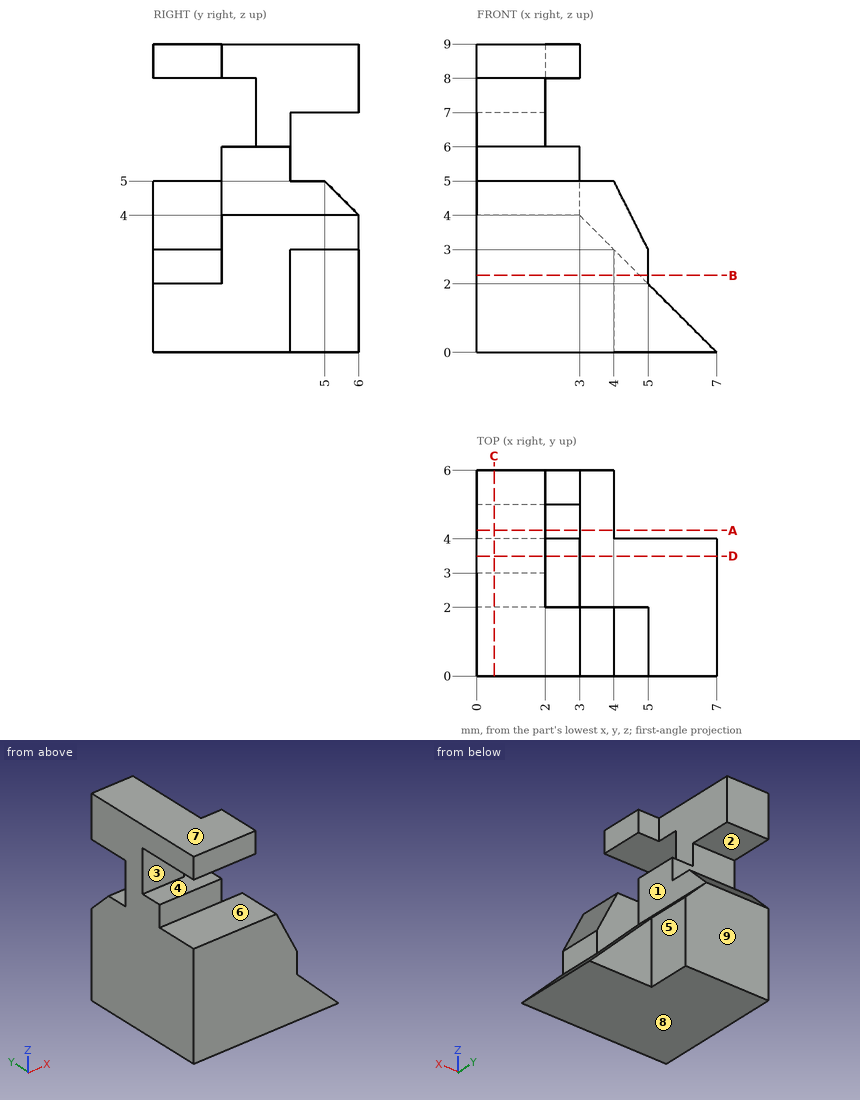
Check sheet for the drawn part. Datum: minimum x, y, z corner. Units: mm. A direction names the side the tool comes from. Round coordinates to 2 decimals unless told otherwise and drop trailing zeros. Loops run counter-clockwise (first coordinate to the right, second up) from the corner with the lowest first, then second, coordinate; pieces in that order, holes last.
Item 1: Thickness scan on line 1 (Z direction, x = 1, y = 0.5); line 2 (Z direction, x = 5, y = 3). Record the ranges inside material, lowest first.
Item 2: Cross-section at A-A on y = 4.25. Record the boundary of the cut face in (x, z), then the cut area to 3 significant figures.
Item 3: Access from +Z, -Z, +X, -X, +Y, -Y to the whole of each face (thin tool, end or side, straight path). Record for the marked faces 1, 2, 3, 4 and 5.
Item 4: Cross-section at C-C on x = 0.5. Record the boundary of the cut face in (y, z).
Item 5: Gauge pin test, flat ends, axial feed: pin 1 (0.5 mm diameter, centred on x = 2.5, z = 8.5, fed in from +Y); pin 2 (0.8 mm diameter, centred on x = 1.5, z = 5.5, fed in from -Y); pin 3 (0.6 mm diameter, centred on x = 2, z = 6.5, fed in from +Y); pin 4 (1.5 mm diameter, centred on x = 0.5, z = 4.5, fed in from +Y). Record the tip position at first contact, or that the pin passes through.
Item 6: Mould release check, pull along Z, two halves, no side actions. Record for the marked faces 6, 7, 8 and 9: pulls with the +Z half, pulls with the -Z half, needs draft (parallel to the pull), parting line crosses it, or undercut.
Item 7: Cross-section at B-B on z = 2.25. Record the boundary of the cut face in (x, y), then the cut area to 3 significant figures.
Item 8: Cross-section at D-D on y = 3.5. Record the boundary of the cut face in (x, z).
Answer sheet:
1. line 1: z = 0 to 5, 8 to 9
1. line 2: z = 0 to 2
2. outline: (0, 0) - (4, 0) - (4, 3) - (3, 4) - (3, 5) - (0, 5) - close; (0, 7) - (2, 7) - (2, 9) - (0, 9) - close
2. area: 22.5 mm2
3. face 1: +Z, +X, +Y
3. face 2: +X, -X, +Y
3. face 3: +X, -X, -Y
3. face 4: +X, -Y
3. face 5: +Z, -Z, +X, +Y
4. outline: (0, 0) - (6, 0) - (6, 4) - (5, 5) - (4, 5) - (4, 7) - (6, 7) - (6, 9) - (0, 9) - (0, 8) - (3, 8) - (3, 6) - (2, 6) - (2, 5) - (0, 5) - close
5. pin 1: stops at y = 2
5. pin 2: stops at y = 2
5. pin 3: stops at y = 4
5. pin 4: stops at y = 6
6. face 6: undercut
6. face 7: pulls with the +Z half
6. face 8: pulls with the -Z half
6. face 9: needs draft
7. outline: (0, 0) - (5, 0) - (5, 2) - (4.75, 2) - (4.75, 4) - (4, 4) - (4, 6) - (0, 6) - close
7. area: 27.5 mm2
8. outline: (0, 0) - (7, 0) - (3, 4) - (3, 6) - (2, 6) - (2, 9) - (0, 9) - close
